Geometry: final body of the model. Coordinates: model frame, mm. Face numbers are marked on the shaded views. Round coordinates to 2 decimals unless told otherwise and drop trailing zeros. Put each result on its own line as item: value. Start each with the question number.
1) Material intervals for probe 1 along X at (y, z) = (-14.5, 8); probe 2 along Z at (x, y) = (76, -10.5); probe 3 along Z at (x, y) = (51.5, 0), sorted ascending. Write a range as [from, to].
2) Draft query along X for the marked faces 1, 2 and 3. Return one class per face: pulls with the +X half, pulls with the -X half, needs draft (parallel to the pull), parting line crosses it, or undercut.
3) First-contact query: P1, Ø4, axis at x = 36.5, y = 4, coming from the +Z side; P2, Ø4, axis at x = 124.5, y = -27, coming from the +Z side; P3, Ø5, axis at x = 43, y = -8, coming from the +Z side. Flat tips, straight axial feed; report the tip coordinate or a pass-through.
from build123d import *

# Parameters (mm, degrees)
IZIM6_R                     = 5
IZIM7_R                     = 7
Y_KSEKLIK_EKSTR_ZYON4_DEPTH = 4
IZIM8_R                     = 9
Y_KSEKLIK_EKSTR_ZYON5_DEPTH = 14
Y_KSEKLIK_EKSTR_ZYON6_DEPTH = 6.8
PAH3_SIZE                   = 1
PAH4_SIZE                   = 3
PAH4_SIZE2                  = 1.732050808
KES_EKSTR_ZYON2_DEPTH       = 40
IZIM16_R                    = 5
KES_EKSTR_ZYON3_DEPTH       = 20
IZIM17_R                    = 4


# Read off the part's stored shape, not the designer's step: Kes-Döndür5
with BuildPart() as part:
    # Süpür2: sweep along a curve in space
    with BuildLine() as s_p_r2_path:
        Line((0, 0, 0), (56.718021516, -1.806734242, 0))
        ThreePointArc((62.272824235, -2.779118041, 0), (59.529866977, -2.096162077, 0), (56.718021516, -1.806734242, 0))
        Line((62.272824235, -2.779118041, 0), (93.753257718, -13.028291116, 0))
        ThreePointArc((112.028316303, -18.42927259, 13.897253926), (105.011429248, -16.541825325, 3.843978082), (93.753257718, -13.028291116, 0))
        Line((112.028316303, -18.42927259, 13.897253926), (127.219469031, -21.476290386, 61.973686406))
    # Çizim6 → Süpür2 (sweep)
    with BuildSketch(Plane(origin=(0, 0, 0), x_dir=(0, 0, -1), z_dir=(0.9994930255797312, -0.03183852725040804, 0))):
        Circle(IZIM6_R)
    sweep(path=s_p_r2_path.line)

    # Çizim7 → Yükseklik-Ekstrüzyon4 (add)
    with BuildSketch(Plane(origin=(0, 0, 0), x_dir=(0, 0, 1), z_dir=(-0.9994930255797312, 0.03183852725040805, 0))):
        with Locations(Location((0, 0, 0), (0, 0, 270))):
            Circle(IZIM7_R)
    extrude(amount=-Y_KSEKLIK_EKSTR_ZYON4_DEPTH)

    # Çizim8 → Yükseklik-Ekstrüzyon5 (add)
    with BuildSketch(Plane(origin=(3.997972102, -0.127354109, 0), x_dir=(0, 0, -1), z_dir=(0.9994930255797312, -0.031838527250408054, 0))):
        with Locations(Location((0, 0, 0), (0, 0, 90))):
            Circle(IZIM8_R)
    extrude(amount=Y_KSEKLIK_EKSTR_ZYON5_DEPTH)

    # Çizim9 → Yükseklik-Ekstrüzyon6 (add)
    with BuildSketch(Plane(origin=(17.99087446, -0.573093491, 0), x_dir=(0, 0, -1), z_dir=(0.9994930255797312, -0.03183852725040806, 0))):
        Polygon((10.969655115, 0), (5.484827557, 9.5), (-5.484827557, 9.5), (-10.969655115, 0), (-5.484827557, -9.5), (5.484827557, -9.5), align=None)
    extrude(amount=Y_KSEKLIK_EKSTR_ZYON6_DEPTH)

    # Pah3
    pah3_edges = [part.edges().sort_by_distance(p)[0] for p in [
        (3.711425357, -9.122791339, 0),
    ]]
    chamfer(pah3_edges, length=PAH3_SIZE)

    # Pah4
    pah4_edges = [part.edges().sort_by_distance(p)[0] for p in [
        (0.222869691, 6.996451179, 0),
    ]]
    pah4_side = [part.faces().sort_by_distance(p)[0] for p in [
        (2.221855742, 6.932774125, 0),
    ]]
    chamfer(pah4_edges, length=PAH4_SIZE, length2=PAH4_SIZE2, reference=pah4_side[0])

    # Çizim10 → Kes-Döndür2 (revolve, cut)
    with BuildSketch(Plane.XY):
        Polygon((22.618780487, 10.827793669), (25.852660243, 7.381106616), (28.637042918, 10.827793669), align=None)
        Polygon((20.847453028, 10.838567795), (17.932722309, 8.103800024), (15.366806113, 10.838567795), align=None)
    revolve(axis=Axis((17.99087446, -0.573093491, 0), (0.9994930255797312, -0.03183852725040806, 0)), mode=Mode.SUBTRACT)

    # Çizim14 → Döndür2 (revolve)
    with BuildSketch(Plane(origin=(29.636413051, -5.944425654, 93.792290583), x_dir=(0.9537039040924367, 0.019022772482439516, -0.30014496072052566), z_dir=(0.30074717508040627, -0.06032340080439443, 0.9517942130505669))):
        with BuildLine():
            Line((102.320076034, -2.513344877), (102.320076034, -32.513344877))
            ThreePointArc((102.320076034, -32.513344877), (117.320076034, -17.513344877), (102.320076034, -2.513344877))
        make_face()
    revolve(axis=Axis((127.219469031, -6.506326297, 62.922462025), (0, -0.9979976059302316, -0.06325170794157503)))

    # Çizim15 → Kes-Ekstrüzyon2 (cut)
    with BuildSketch(Plane(origin=(0, 0, 0), x_dir=(1, 0, 0), z_dir=(0, 1, 0))):
        Polygon((132.389771245, -43.488442314), (142.340651861, -78.720795845), (151.231048207, -76.209828969), (141.280167591, -40.977475439), align=None)
        Polygon((113.00322211, -48.430617202), (123.048070303, -83.99567484), (112.182017345, -87.064638021), (102.137169152, -51.499580383), align=None)
    extrude(amount=-KES_EKSTR_ZYON2_DEPTH, mode=Mode.SUBTRACT)

    # Çizim16 → Kes-Ekstrüzyon3 (cut)
    with BuildSketch(Plane(origin=(91.986882531, 0, -25.980395705), x_dir=(0.2718029884745819, 0, 0.9623529162715133), z_dir=(-0.9623529162715133, 0, 0.2718029884745819))):
        with Locations((94.21918972, -21.476290386)):
            Circle(IZIM16_R)
    extrude(amount=-KES_EKSTR_ZYON3_DEPTH, mode=Mode.SUBTRACT)

    # Kes-Süpür2: sweep along a curve in space
    with BuildLine() as kes_s_p_r2_path:
        Line((0, 0, 0), (56.718021516, -1.806734242, 0))
        ThreePointArc((62.272824235, -2.779118041, 0), (59.529866977, -2.096162077, 0), (56.718021516, -1.806734242, 0))
        Line((62.272824235, -2.779118041, 0), (93.753257718, -13.028291116, 0))
        ThreePointArc((112.028316303, -18.42927259, 13.897253926), (105.011429248, -16.541825325, 3.843978082), (93.753257718, -13.028291116, 0))
        Line((112.028316303, -18.42927259, 13.897253926), (127.219469031, -21.476290386, 61.973686406))
    # Çizim17 → Kes-Süpür2 (sweep, cut)
    with BuildSketch(Plane(origin=(0, 0, 0), x_dir=(0, 0, 1), z_dir=(-0.9994930255797312, 0.03183852725040805, 0))):
        Circle(IZIM17_R)
    sweep(path=kes_s_p_r2_path.line, mode=Mode.SUBTRACT)

    # Kes-Döndür5 outline → Kes-Döndür5 (revolve, cut)
    with BuildSketch(Plane(origin=(25.609057337, -21.476290386, 90.672111995), x_dir=(0, 1, 0), z_dir=(-0.2718029884745821, 0, -0.9623529162715133))):
        with BuildLine():
            ThreePointArc((5, 101.687958803), (8.1, 105.585393857), (5, 109.482828911))
            Line((5, 109.482828911), (5, 101.687958803))
        make_face()
    revolve(axis=Axis((25.609057337, -21.476290386, 90.672111995), (0.9623529162715133, 0, -0.2718029884745821)), mode=Mode.SUBTRACT)


solid = part.part
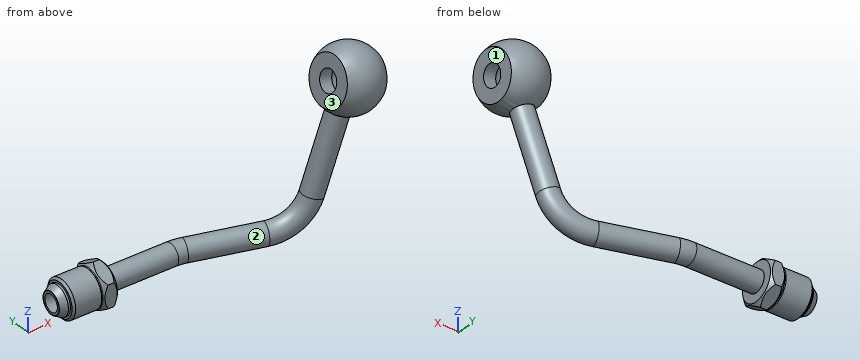
Result sheet:
1. probe 1: x = [103.05, 105.19], [111.66, 113.34]
1. probe 2: z = [-3.93, -2.54], [2.54, 3.93]
1. probe 3: z = [-4.72, -3.65], [3.65, 4.72]
2. face 1: pulls with the +X half
2. face 2: undercut
2. face 3: pulls with the -X half
3. P1: stops at z = 3.87
3. P2: stops at z = 76.39
3. P3: stops at z = 2.82
